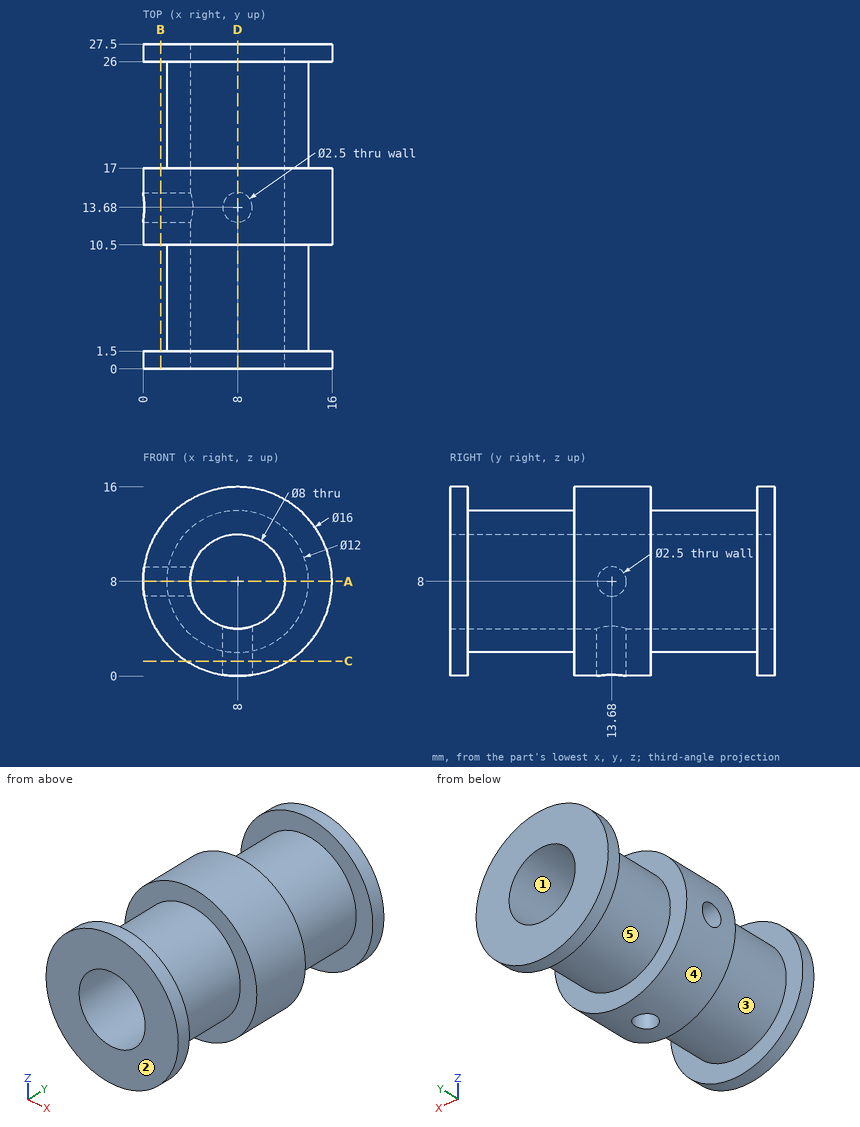
The drawing under review shows one solid part. Ordinate dimensions are in mm from its lowest x, y, z. A direction names the side the tool comes from. Coordinates: 2 decimals unless noted, no trailing zeros. Write each loop counter-clockwise with the first axis right and the second up, starting at its lowest first coordinate (ties: lowest second). Pieces come first, ordered by that corner, then holes. Notation, with made-up numbers: (-1, 41) - (24, 41) arc R27 cw to (24, 80) - close; hole circle Ø5 at (82, 80). An arc over 180 degrees is marked (long way). Answer in a Markdown table with one row per item. Add a question column.
Q1. We need section D-D, the plane x = 8. State the section outline as (y, z) points.
Q2. Tool access review of the marked faces 4 and 5: name each direction out of +Z, -Z, +X, -X, +Y, -Y from which nothing blocks a thin tool from reaching the whole face with its end or side.
Q3. We need section C-C, the plane z = 1.25. State the section outline as (x, y) points, and give its area (3 significant figures).
Q4. For probe 1 along Y at (x, z) = (2.5, 2.25); probe 2 along Y at (x, z) = (8, 1.8); probe 3 along Y at (x, z) = (8, 2.35), list the stretches that pass through material, from the lowest coordinate up.
Q5. We need section B-B, the plane x = 1.5. State the section outline as (y, z) points.
Q6. We need section A-A, the plane z = 8. State the section outline as (x, y) points, and give its area (3 significant figures).
Q7. For P1, Ø1, axis at y = 4, z = 6, coming from the +X side; P2, Ø5, axis at x = 9, z = 7, coming from the -Y side (3 decimals); P3, Ø1.5, axis at y = 8, z = 12.5, coming from the +X side; P4, Ø3, axis at y = 14.5, z = 12.5, coming from the +X side, all flat-tipped, find the tip position at first contact; note any pin that passes through.
Q8. Draft analysis for pull direction X (two halves, no side actions). For the marked faces 1, 2 and 3, state which applies: +X half, -X half, draft (parallel to the pull), parting line (faces both ways), or undercut.
Answer list:
| question | item | result |
|---|---|---|
| 1 | outline | (0, 0) - (1.5, 0) - (1.5, 2) - (10.5, 2) - (10.5, 0) - (12.43, 0) - (12.43, 4) - (0, 4) - close; (0, 12) - (27.5, 12) - (27.5, 16) - (26, 16) - (26, 14) - (17, 14) - (17, 16) - (10.5, 16) - (10.5, 14) - (1.5, 14) - (1.5, 16) - (0, 16) - close; (14.93, 0) - (17, 0) - (17, 2) - (26, 2) - (26, 0) - (27.5, 0) - (27.5, 4) - (14.93, 4) - close |
| 2 | face 4 | +Y, -Y |
| 2 | face 5 | none |
| 3 | outline | (3.71, 0) - (12.29, 0) - (12.29, 1.5) - (3.71, 1.5) - close; (3.71, 10.5) - (12.29, 10.5) - (12.29, 17) - (3.71, 17) - close; (3.71, 26) - (12.29, 26) - (12.29, 27.5) - (3.71, 27.5) - close; hole circle Ø2.5 at (8, 13.68) |
| 3 | area | 76.7 mm2 |
| 4 | probe 1 | y = 0 to 1.5, 10.5 to 17, 26 to 27.5 |
| 4 | probe 2 | y = 0 to 1.5, 10.5 to 12.43, 14.93 to 17, 26 to 27.5 |
| 4 | probe 3 | y = 0 to 12.43, 14.93 to 27.5 |
| 5 | outline | (0, 3.34) - (1.5, 3.34) - (1.5, 12.66) - (0, 12.66) - close; (10.5, 3.34) - (17, 3.34) - (17, 12.66) - (10.5, 12.66) - close; (26, 3.34) - (27.5, 3.34) - (27.5, 12.66) - (26, 12.66) - close; hole circle Ø2.5 at (13.68, 8) |
| 6 | outline | (0, 0) - (4, 0) - (4, 12.43) - (0, 12.43) - (0, 10.5) - (2, 10.5) - (2, 1.5) - (0, 1.5) - close; (0, 14.93) - (4, 14.93) - (4, 27.5) - (0, 27.5) - (0, 26) - (2, 26) - (2, 17) - (0, 17) - close; (12, 0) - (16, 0) - (16, 1.5) - (14, 1.5) - (14, 10.5) - (16, 10.5) - (16, 17) - (14, 17) - (14, 26) - (16, 26) - (16, 27.5) - (12, 27.5) - close |
| 6 | area | 138 mm2 |
| 7 | P1 | stops at x = 13.81 |
| 7 | P2 | passes through |
| 7 | P3 | stops at x = 12.68 |
| 7 | P4 | stops at x = 15.42 |
| 8 | face 1 | undercut |
| 8 | face 2 | draft |
| 8 | face 3 | parting line |
